```python
from build123d import *

# Parameters (mm, degrees)
F0_W     = 213.36
F0_H     = 146.05
F1_DEPTH = 1.5748
F2_W     = 205.2828
F2_H     = 143.51
F3_DEPTH = 1.778


with BuildPart() as f1:
    # F0 (on Front) → F1 (new body, symmetric)
    with BuildSketch(Plane.XZ):
        Rectangle(F0_W, F0_H)
    extrude(amount=F1_DEPTH, both=True)

    # F2 (on face) → F3 (cut)
    with BuildSketch(Plane(origin=(0, 1.5748, 0), x_dir=(-1, 0, 0), z_dir=(0, 1, 0))):
        with Locations((-0.084434, 1.27)):
            Rectangle(F2_W, F2_H)
    extrude(amount=-F3_DEPTH, mode=Mode.SUBTRACT)


solid = f1.part
```
Geometry check sheet. Reference: the model listing, model coordinates, mm. Round coordinates to 2 decimals unless told otherwise and drop trailing zeros. Loops run counter-clockwise (first coordinate to the right, second up) from the corner with the lowest first, then second, coordinate; pieces in that order, holes last. Notation, with made-up numbers: (-2, 51.25) - (49, 51.25) arc R33 ccw to (49, 83.25) - close; hole circle Ø6 at (-1, 28). An arc over 180 degrees is marked (long way). Use a Markdown table: item, result.
Q1. Go/stop test with a flat-tipped pin: P1, Ø0.9, axis at x = -18, y = 0.5, coming from the +Z side (3 decimals). Record where the tip stops, or that it passes through.
Solutions:
| item | result |
|---|---|
| P1 | stops at z = -70.485 |
Q2. Material ranges on line 1 (X direction, y = 1.35, z = 15); line 2 (Y direction, x = -75, z = -57); line 3 (Z direction, x = -47, y = 0.9) (3 decimals), recorded low to high.
Solutions:
| item | result |
|---|---|
| line 1 | x = -106.68 to -102.56, 102.73 to 106.68 |
| line 2 | y = -1.57 to -0.2 |
| line 3 | z = -73.025 to -70.485 |
Q3. Cross-section at B-B on x = -82. Record the cut outline in (y, z) (3 decimals), plus the area to 3 significant figures.
Solutions:
| item | result |
|---|---|
| outline | (-1.575, -73.025) - (1.575, -73.025) - (1.575, -70.485) - (-0.203, -70.485) - (-0.203, 73.025) - (-1.575, 73.025) - close |
| area | 205 mm2 |
Q4. Cross-section at A-A on y = 0.9. Record the cut outline in (x, z) (3 decimals).
Solutions:
| item | result |
|---|---|
| outline | (-106.68, -73.025) - (106.68, -73.025) - (106.68, 73.025) - (102.726, 73.025) - (102.726, -70.485) - (-102.557, -70.485) - (-102.557, 73.025) - (-106.68, 73.025) - close |
Q5. Cross-section at C-C on z = -2.5. Record the cut outline in (x, y), plus the area to 3 significant figures.
Solutions:
| item | result |
|---|---|
| outline | (-106.68, -1.57) - (106.68, -1.57) - (106.68, 1.57) - (102.73, 1.57) - (102.73, -0.2) - (-102.56, -0.2) - (-102.56, 1.57) - (-106.68, 1.57) - close |
| area | 307 mm2 |
Q6. Draft check along X on faces 1 (the flat face through (-1, -1.575, 1)), 2 (the flat face through (2, -0.203, 2)). Enter one of: released by +X, released by -X, zero draft, split by the parting line, or undercut.
Solutions:
| item | result |
|---|---|
| face 1 | zero draft |
| face 2 | undercut |
